Could you check a few things on this model? Use its own coordinates, in mm. Face numbers are marked on the shaded views. A direction names the side the tool comes from. Give positions to 0.01 mm unless a question says otherwise; leave off trailing zeros. Loops run counter-clockwise (first coordinate to the right, second up) from the corner with the lowest first, then second, coordinate; pieces in that order, holes last. Notation, with made-up numbers: M 48,85 L 68,85 A24 cw 68,116 Z; hole C 24.25,87 d11. An arc over 180 degrees is marked long. Use a Markdown table: item, result. Add a question column.
1) Will these pins go through, and if not, where does the flat tip stop? pin 1 Ø1 at (y, z) = (15, 18) entering from +X; pin 2 Ø9 at (y, z) = (19.5, 38.5) entering from -X; pin 3 Ø4 at (y, z) = (16.5, 32) entering from +X; pin 4 Ø1 at (y, z) = (8.5, 6.5) entering from +X.
2) Suppose I cut it at D-D on x = -14. List the corners of the cut face in (y, z) for me, and give its area (3 significant figures).
3) If I drill on line 1 along Y through (x, z) = (-25, 46.5); line 2 along Z through (x, y) = (-22.5, 10); line 3 along Z through (x, y) = (-6.5, 13), over which ranges is the centre line in solid material (lowest first)? Write a range as [from, to].
4) Suppose I cut it at B-B on y = 21.3. List the corners of the cut face in (x, z) for me.
5) Suppose I cut it at C-C on z = 33.5. List the corners of the cut face in (x, y) for me.
6) Suppose I cut it at A-A on x = -20. List the corners of the cut face in (y, z) for me, and give its area (3 significant figures).
7) We'd pull the mould along Z, two halves only. Please class the marked faces 1, 2 and 3: +Z half, -Z half, draft (parallel to the pull), parting line (faces both ways), or undercut.
8) Which directions (+Z, -Z, +X, -X, +Y, -Y) give clear straight access to the entire face, cutting with the end or side of a thin tool? Please do the marked faces 4, 5, 6 and 7.
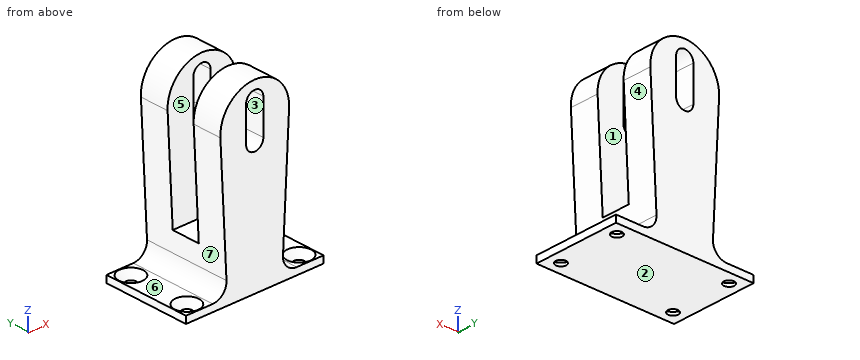
Autodesk Inventor part; units mm, degrees
ref_plane "YZ Plane" through (0, 0, 0) normal (1, 0, 0) x (0, 1, 0)
ref_plane "XZ Plane" through (0, 0, 0) normal (0, 1, 0) x (-1, 0, 0)
ref_plane "XY Plane" through (0, 0, 0) normal (0, 0, 1) x (1, 0, 0)
sketch "Skizze3" plane through (0, 0, 0) normal (0, 0, 1) x (1, 0, 0)
  line L0 (0, 0) -> (-40, 0)
  line L1 (-40, 0) -> (-40, 25)
  line L2 (-40, 25) -> (0, 25)
  line L3 (0, 25) -> (0, 0)
  point P0 (-3.7, 3.7)
  dimension "d4" = 25
  dimension "d5" = 40
  dimension "d6" = 3.7
  dimension "d7" = 3.7
sketch "Skizze4" plane through (0, 0, 0) normal (0, 1, 0) x (-1, 0, 0)
  line L0 (0, 0) -> (40, 0)
  line L1 (20, 0) -> (20, 50)
  line L2 (20, 45) -> (20, 35) construction
  line L3 (22.5, 45) -> (22.5, 35)
  line L4 (17.5, 35) -> (17.5, 45)
  arc A0 (22.5, 45) -> (17.5, 45) centre (20, 45) ccw
  arc A1 (17.5, 35) -> (22.5, 35) centre (20, 35) ccw
  circle A2 centre (20, 40) radius 10
  line L5 (29.9874, 39.4975) -> (28, 0)
  line L6 (10.0126, 39.4975) -> (12, 0)
  dimension "d8" = 50
  dimension "d9" = 10
  dimension "d10" = 5
  dimension "d11" = 10
  dimension "d12" = 8
  dimension "d13" = 8
extrude "Extrusion3" add sketch "Skizze4" along normal blind 25 contours L6 A2 L1 L0 | L1 A2 L5 L0 | A2 L1 A0 L4 A1 | L1 A1 L3 A0 A2
extrude "Extrusion4" add sketch "Skizze3" against normal blind 2
hole "Bohrung1" at (-3.7, 3.7, 0) direction (0, 0, -1) diameter 2.459 depth 8.8 countersink diameter 7 countersink angle 90
sketch "Skizze5" plane through (0, 0, 0) normal (1, 0, 0) x (0, 0, -1)
  line L0 (-50, 0) -> (-50, 25)
  line L1 (-50, 8.4) -> (-10, 8.4)
  line L2 (-10, 8.4) -> (-10, 16.6)
  line L3 (-10, 16.6) -> (-50, 16.6)
  line L4 (-50, 16.6) -> (-50, 8.4)
  point P0 (0, 0)
  point P1 (-50, 12.5)
  dimension "d25" = 8.2
  dimension "d26" = 40
extrude "Extrusion5" cut sketch "Skizze5" against normal through all
pattern_linear "Rechteckige Anordnung1" count 2 spacing 32.6 along (-1, 0, 0) count 2 spacing 17.6 along (0, 1, 0) of "Bohrung1"
fillet "Rundung1" radius 4 2 edges at (-28, 12.5, 0) (-12, 12.5, 0)
equation "\"d13\" = d12"
equation "\"d14\" = d4"
equation "\"d31\" = d5 - 2 * d6"
equation "\"d34\" = d4 - 2 * d7"
properties part number "BT101_trajan20_21"
Answer block:
| question | item | result |
|---|---|---|
| 1 | pin 1 | passes through |
| 1 | pin 2 | stops at x = -30 |
| 1 | pin 3 | stops at x = -10.29 |
| 1 | pin 4 | stops at x = -11.65 |
| 2 | outline | M 0,-2 L 25,-2 L 25,48 L 16.6,48 L 16.6,10 L 8.4,10 L 8.4,48 L 0,48 Z |
| 2 | area | 938 mm^2 |
| 3 | line 1 | y = [0, 8.4], [16.6, 25] |
| 3 | line 2 | z = [-2, 10] |
| 3 | line 3 | z = [-2, 0] |
| 4 | outline | M -40,-2 L -37.8,-2 L -39.8,0 L -40,0 Z; M -34.8,-2 L -5.2,-2 L -7.2,0 L -7.79,0 A4 cw -11.79,4.2 L -10.01,39.5 A10 ccw long -29.99,39.5 L -28.21,4.2 A4 cw -32.21,0 L -32.8,0 Z; M -2.2,-2 L 0,-2 L 0,0 L -0.2,0 Z; hole M -22.5,35 A2.5 ccw -17.5,35 L -17.5,45 A2.5 ccw -22.5,45 Z |
| 5 | outline | M -29.69,0 L -22,0 L -22,8.4 L -29.69,8.4 Z; M -29.69,16.6 L -22,16.6 L -22,25 L -29.69,25 Z; M -18,0 L -10.31,0 L -10.31,8.4 L -18,8.4 Z; M -18,16.6 L -10.31,16.6 L -10.31,25 L -18,25 Z |
| 6 | outline | M 0,-2 L 25,-2 L 25,32.5 L 16.6,32.5 L 16.6,10 L 8.4,10 L 8.4,32.5 L 0,32.5 Z; M 0,47.5 L 8.4,47.5 L 8.4,50 L 0,50 Z; M 16.6,47.5 L 25,47.5 L 25,50 L 16.6,50 Z |
| 6 | area | 720 mm^2 |
| 7 | face 1 | draft |
| 7 | face 2 | -Z half |
| 7 | face 3 | undercut |
| 8 | face 4 | +X, +Y, -Y |
| 8 | face 5 | +Z, +X, -X |
| 8 | face 6 | +Z, -X, +Y, -Y |
| 8 | face 7 | -X, +Y, -Y |
